Geometry: final body of the model. Coordinates: model frame, mm. Face numbers are marked on the shaded views. A direction names the side the tool comes from. Coordinates: 2 decimals unless noted, no trailing zeros. Order: outer loops, then holes, each group sorted by start corner. A loop starts at its lowest first (then second) coordinate and runs counter-clockwise, first axis right, second up. Notation, with made-up numbers: M -1,33 L 35,33 A13 cw 35,49 Z; hole C -4,61.25 d1. An arc over 180 degrees is marked long. One line per question, with ' | ' between items.
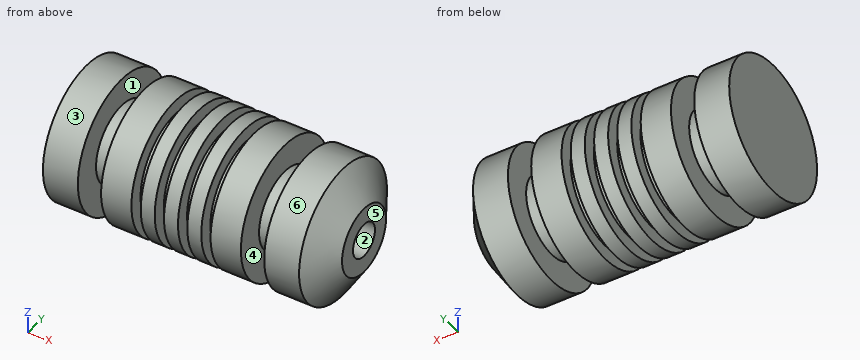
from build123d import *

# Parameters (mm, degrees)
SKETCH3_R          = 3.81
CUT_EXTRUDE1_DEPTH = 2.54
CUT_EXTRUDE1_TAPER = 56


with BuildPart() as part:
    # Sketch1 → Revolve5 (revolve)
    with BuildSketch(Plane.XY):
        Polygon((0, 0), (113.03, 0), (113.03, 3.81), (125.73, 3.81), (125.73, 6.35), (138.43, 6.35), (138.43, 9.2075), (151.13, 9.2075), (151.13, 18.415), (139.700007257, 36.83), (120.650007257, 36.83), (120.650007257, 21.59), (107.950007257, 21.59), (107.950007257, 36.83), (91.440007257, 36.83), (91.440007257, 29.21), (86.360007257, 29.21), (86.360007257, 36.83), (78.740007257, 36.83), (78.740007257, 29.21), (73.660007257, 29.21), (73.660007257, 36.83), (66.040007257, 36.83), (66.040007257, 29.21), (60.960007257, 29.21), (60.960007257, 36.83), (53.340007257, 36.83), (53.340007257, 29.21), (48.260007257, 29.21), (48.260007257, 36.83), (31.750007257, 36.83), (31.750007257, 21.59), (19.050007257, 21.59), (19.050007257, 36.83), (0, 36.83), align=None)
    revolve(axis=Axis((0, 0, 0), (1, 0, 0)))

    # Sketch3 → Cut-Extrude1 (cut)
    with BuildSketch(Plane(origin=(113.03, 0, 0), x_dir=(0, 0, -1), z_dir=(1, 0, 0))):
        Circle(SKETCH3_R)
    extrude(amount=-CUT_EXTRUDE1_DEPTH, taper=CUT_EXTRUDE1_TAPER, mode=Mode.SUBTRACT)


solid = part.part
1. Section B-B, the plane z = -31. Give the number of separate pieces and of enclosed holes in the cut face, and give its area (3 significant figures).
Response values:
separate pieces: 7 | enclosed holes: 0 | area: 3,830 mm^2
2. Section A-A, the plane x = 41. Output: boundary loops of the cut face in (y, z).
Response values:
outline: C 0,0 d73.66
3. Draft query along X for the marked faces 4, 5 and 6. Return one class per face: pulls with the +X half, pulls with the -X half, needs draft (parallel to the pull), parting line crosses it, or undercut.
Response values:
face 4: undercut | face 5: pulls with the +X half | face 6: needs draft
4. Pin query (flat end, axial travel): P1, Ø3, axis at y = -25.5, z = -1.5, coming from the +X side; P2, Ø4, axis at y = -1, z = -2, coming from the +X side; P3, Ø3, axis at x = 69.5, y = 7.5, coming from the +Z side. Return the tip coordinate at first contact, or that it passes through.
Response values:
P1: stops at x = 147.64 | P2: stops at x = 125.73 | P3: stops at z = 36.34
5. Access query for the marked faces 1, 2 and 3. Directions: +Z, -Z, +X, -X, +Y, -Y. A direction counts if a zero-diameter tool reaches every point of the face in a straight line with its end or side. Return the directions, or none.
Response values:
face 1: none | face 2: +X | face 3: +X, -X
6. Section C-C, the plane x = 123. Output: boundary loops of the cut face in (y, z).
Response values:
outline: C 0,0 d73.66; hole C 0,0 d7.62
7. Material intervals for line 1 (Z direction, x = 128.75, y = 0); line 2 (X direction, y = 6.5, z = -25.5); line 3 (X direction, y = -23, z = -13.5), sorted ascending. Write a range as [from, to].
Response values:
line 1: z = [-36.83, -6.35], [6.35, 36.83] | line 2: x = [0, 19.05], [31.75, 107.95], [120.65, 146.23] | line 3: x = [0, 19.05], [31.75, 107.95], [120.65, 146.01]
